The listing builds one solid part. Answer for the finished solid, in the listing's coordinates (mm). Face numbers are marked on the shaded views. A direction names the side the tool comes from. Round coordinates to 2 decimals unless told otherwise and drop trailing zeros. Loops run counter-clockwise (first coordinate to the right, second up) from the corner with the lowest first, then second, coordinate; pieces in that order, holes last. Notation, with made-up numbers: M -12.75,-19.5 L 5.25,-19.5 A32 cw 5.25,19.5 Z; hole C -18.5,19 d6. An arc over 180 degrees is marked long. Answer as a JSON object with one key per item and string values.
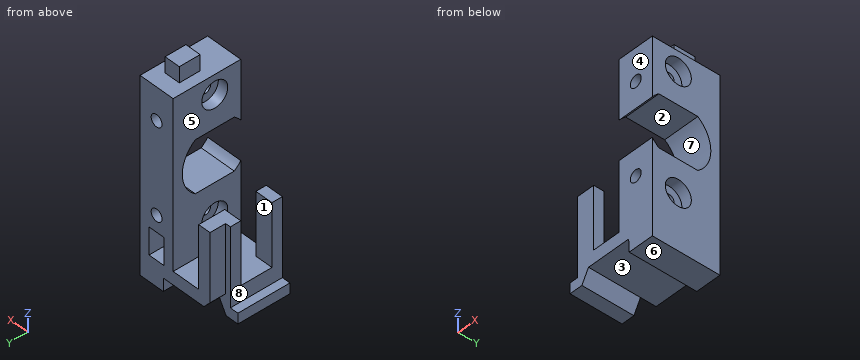
```python
from build123d import *

# Parameters (mm, degrees)
SKETCH2_R           = 1
BOSS_EXTRUDE1_DEPTH = 7
CUT_EXTRUDE1_START  = -5
SKETCH3_R           = 1.15
CUT_EXTRUDE1_DEPTH  = 13
SKETCH5_R           = 2.5
CUT_EXTRUDE2_DEPTH  = 2
CUT_EXTRUDE3_START  = 7
SKETCH5_2_R         = 2.5
CUT_EXTRUDE3_DEPTH  = 2
BOSS_EXTRUDE2_START = -5
BOSS_EXTRUDE2_DEPTH = 13
CUT_EXTRUDE4_START  = -5.4
SKETCH7_W           = 12
SKETCH7_H           = 6
CUT_EXTRUDE4_DEPTH  = 5
CUT_EXTRUDE5_START  = -10.4
SKETCH8_W           = 15
SKETCH8_H           = 13
CUT_EXTRUDE5_DEPTH  = 1.6
CUT_EXTRUDE6_START  = -8.8
SKETCH9_W           = 13
SKETCH9_H           = 3
CUT_EXTRUDE6_DEPTH  = 1
BOSS_EXTRUDE4_START = 8
SKETCH10_W          = 5.4
SKETCH10_H          = 5
BOSS_EXTRUDE4_DEPTH = 13
CUT_EXTRUDE7_START  = 8
SKETCH11_W          = 17.4
SKETCH11_H          = 3
CUT_EXTRUDE7_DEPTH  = 13
BOSS_EXTRUDE5_START = 15
SKETCH12_W          = 3
SKETCH12_H          = 4
BOSS_EXTRUDE5_DEPTH = 3
CUT_EXTRUDE8_START  = 8
CUT_EXTRUDE8_DEPTH  = 13
CUT_EXTRUDE9_START  = 8
CUT_EXTRUDE9_DEPTH  = 3
CUT_EXTRUDE10_START = 8
SKETCH15_W          = 3.2
SKETCH15_H          = 5.2
CUT_EXTRUDE10_DEPTH = 3.2


with BuildPart() as part:
    # Sketch2 → Boss-Extrude1 (new body)
    with BuildSketch(Plane(origin=(0, 0, 0), x_dir=(0, 0, -1), z_dir=(1, 0, 0))):
        with BuildLine():
            Line((3.75, -5), (15, -5))
            Line((15, -5), (15, 8))
            Line((15, 8), (-15, 8))
            Line((-15, 8), (-15, -5))
            Line((-15, -5), (-3.75, -5))
            ThreePointArc((-3.75, -5), (-4.419417382, -4.419417382), (-5, -3.75))
            Line((-5, -3.75), (-5, 3.75))
            ThreePointArc((-5, 3.75), (0, 6.25), (5, 3.75))
            Line((5, 3.75), (5, -3.75))
            ThreePointArc((5, -3.75), (4.419417382, -4.419417382), (3.75, -5))
        make_face()
        with Locations((-11.25, 0)):
            Circle(SKETCH2_R, mode=Mode.SUBTRACT)
        with Locations((11.25, 0)):
            Circle(SKETCH2_R, mode=Mode.SUBTRACT)
    extrude(amount=BOSS_EXTRUDE1_DEPTH)

    # Sketch3 → Cut-Extrude1 (cut)
    with BuildSketch(Plane(origin=(0, 0, 0), x_dir=(1, 0, 0), z_dir=(0, 1, 0)).offset(CUT_EXTRUDE1_START)):
        with Locations((3.5, 8.75)):
            Circle(SKETCH3_R)
        with Locations((3.5, -8.75)):
            Circle(SKETCH3_R)
    extrude(amount=CUT_EXTRUDE1_DEPTH, mode=Mode.SUBTRACT)

    # Sketch5 → Cut-Extrude2 (cut)
    with BuildSketch(Plane(origin=(0, 0, 0), x_dir=(0, 0, -1), z_dir=(1, 0, 0))):
        with Locations((11.25, 0)):
            Circle(SKETCH5_R)
        with Locations((-11.25, 0)):
            Circle(SKETCH5_R)
    extrude(amount=CUT_EXTRUDE2_DEPTH, mode=Mode.SUBTRACT)

    # Sketch5<2> → Cut-Extrude3 (cut)
    with BuildSketch(Plane(origin=(0, 0, 0), x_dir=(0, 0, -1), z_dir=(1, 0, 0)).offset(CUT_EXTRUDE3_START)):
        with Locations((11.25, 0)):
            Circle(SKETCH5_2_R)
        with Locations((-11.25, 0)):
            Circle(SKETCH5_2_R)
    extrude(amount=-CUT_EXTRUDE3_DEPTH, mode=Mode.SUBTRACT)

    # Sketch6 → Boss-Extrude2 (add)
    with BuildSketch(Plane(origin=(0, 0, 0), x_dir=(1, 0, 0), z_dir=(0, 1, 0)).offset(BOSS_EXTRUDE2_START)):
        Polygon((7, 15), (7, 25), (-10.4, 25), (-10.4, 5), (-5.4, 5), (-5.4, 22), (0, 22), (0, 15), align=None)
    extrude(amount=BOSS_EXTRUDE2_DEPTH)

    # Sketch7 → Cut-Extrude4 (cut)
    with BuildSketch(Plane(origin=(0, 0, 0), x_dir=(0, 0, -1), z_dir=(1, 0, 0)).offset(CUT_EXTRUDE4_START)):
        with Locations((11, 0)):
            Rectangle(SKETCH7_W, SKETCH7_H)
    extrude(amount=-CUT_EXTRUDE4_DEPTH, mode=Mode.SUBTRACT)

    # Sketch8 → Cut-Extrude5 (cut)
    with BuildSketch(Plane(origin=(0, 0, 0), x_dir=(0, 0, -1), z_dir=(1, 0, 0)).offset(CUT_EXTRUDE5_START)):
        with Locations((12.5, 1.5)):
            Rectangle(SKETCH8_W, SKETCH8_H)
    extrude(amount=CUT_EXTRUDE5_DEPTH, mode=Mode.SUBTRACT)

    # Sketch9 → Cut-Extrude6 (cut)
    with BuildSketch(Plane(origin=(0, 0, 0), x_dir=(0, 0, -1), z_dir=(1, 0, 0)).offset(CUT_EXTRUDE6_START)):
        with Locations((11.5, 6.5)):
            Rectangle(SKETCH9_W, SKETCH9_H)
    extrude(amount=CUT_EXTRUDE6_DEPTH, mode=Mode.SUBTRACT)

    # Sketch10 → Boss-Extrude4 (add)
    with BuildSketch(Plane(origin=(0, 0, 0), x_dir=(1, 0, 0), z_dir=(0, 1, 0)).offset(BOSS_EXTRUDE4_START)):
        with Locations((-2.7, 19.5)):
            Rectangle(SKETCH10_W, SKETCH10_H)
    extrude(amount=-BOSS_EXTRUDE4_DEPTH)

    # Sketch11 → Cut-Extrude7 (cut)
    with BuildSketch(Plane(origin=(0, 0, 0), x_dir=(1, 0, 0), z_dir=(0, 1, 0)).offset(CUT_EXTRUDE7_START)):
        with Locations((-1.7, 23.5)):
            Rectangle(SKETCH11_W, SKETCH11_H)
    extrude(amount=-CUT_EXTRUDE7_DEPTH, mode=Mode.SUBTRACT)

    # Sketch12 → Boss-Extrude5 (add)
    with BuildSketch(Plane.XY.offset(BOSS_EXTRUDE5_START)):
        with Locations((3.5, 3)):
            Rectangle(SKETCH12_W, SKETCH12_H)
    extrude(amount=BOSS_EXTRUDE5_DEPTH)

    # Sketch13 → Cut-Extrude8 (cut)
    with BuildSketch(Plane(origin=(0, 0, 0), x_dir=(1, 0, 0), z_dir=(0, 1, 0)).offset(CUT_EXTRUDE8_START)):
        Polygon((2.1, 22), (2.000079904, 19.501997603), (-6.499920096, 19.501997603), (-7.9, 22), align=None)
    extrude(amount=-CUT_EXTRUDE8_DEPTH, mode=Mode.SUBTRACT)

    # Sketch14 → Cut-Extrude9 (cut)
    with BuildSketch(Plane(origin=(0, 0, 0), x_dir=(1, 0, 0), z_dir=(0, 1, 0)).offset(CUT_EXTRUDE9_START)):
        Polygon((-6.499920096, 19.501997603), (-7.8, 18), (-8.8, 18), (-8.8, 20), (-10.4, 20), (-10.4, 22), (-7.9, 22), align=None)
    extrude(amount=-CUT_EXTRUDE9_DEPTH, mode=Mode.SUBTRACT)

    # Sketch15 → Cut-Extrude10 (cut)
    with BuildSketch(Plane(origin=(0, 0, 0), x_dir=(1, 0, 0), z_dir=(0, 1, 0)).offset(CUT_EXTRUDE10_START)):
        with Locations((3.5, 14.5)):
            Rectangle(SKETCH15_W, SKETCH15_H)
    extrude(amount=-CUT_EXTRUDE10_DEPTH, mode=Mode.SUBTRACT)


solid = part.part
```
Item 1: The part is cut by section D-D (z = 8). Give the vertices of the cut face in (x, y).
Values follow:
{"outline": "M 0,-5 L 2.63,-5 L 2.63,8 L 0,8 Z; M 4.37,-5 L 7,-5 L 7,8 L 4.37,8 Z"}
Item 2: Determine the mould class of the marked faces 6, 7 and 8 for opening direction Z: released by +Z, released by -Z, zero draft, split by the parting line, or undercut.
Values follow:
{"face 6": "released by -Z", "face 7": "undercut", "face 8": "zero draft"}
Item 3: Which of the six approach directions +Z, -Z, +X, -X, +Y, -Y give full straight-line access (tool end or side, diameter ignored) to the marked faces 1, 2, 3, 4 and 5?
Values follow:
{"face 1": "+Z, -X", "face 2": "+X, -X", "face 3": "-Z, +Y, -Y", "face 4": "+Z, -Z, +X, -X, -Y", "face 5": "+Z, +Y, -Y"}
Item 4: The part is cut by section A-A (y = -1.5). Give the number of separate pieces and of enclosed holes in the cut face, then the cut area to 3 significant figures.
Values follow:
{"separate pieces": "2", "enclosed holes": "2", "area": "173 mm^2"}
Item 5: The part is cut by section C-C (z = -11.25). Give the vertices of the cut face in (x, y), then the cut area to 3 significant figures.
Values follow:
{"outline": "M -8.8,-5 L -5.4,-5 L -5.4,-3 L -8.8,-3 Z; M -8.8,3 L -5.4,3 L -5.4,8 L -7.8,8 L -7.8,5 L -8.8,5 Z; M 0,-5 L 7,-5 L 7,-2.5 L 5,-2.5 L 5,-1 L 2,-1 L 2,-2.5 L 0,-2.5 Z; M 0,2.5 L 2,2.5 L 2,1 L 5,1 L 5,2.5 L 7,2.5 L 7,8 L 0,8 Z", "area": "85.8 mm^2"}
Item 6: Flat-ended cylindrical pins translate along their axes: P1, Ø6, axis at x = -5, y = -1.5, coming from the +Z side; P2, Ø5.5, axis at y = 1, z = -11.5, coming from the -X side; P3, Ø3, axis at y = 0, z = -11.25, coming from the +X side. Find the tip coordinate at first contact, or state that the pin passes through.
Values follow:
{"P1": "z = -5", "P2": "x = -8.8", "P3": "x = 5"}
Item 7: Straight lines are drawn through the part: line 1 (Z direction, x = 3.65, y = 0); line 2 (Z direction, x = 3.5, y = 2); line 3 (Y direction, x = 5.7, z = 11.25). For each, find the intervals that lie inside material, in ascending order.
Values follow:
{"line 1": "-22 to -12.25, -10.25 to -9.89, -7.61 to -5, 5 to 7.61, 9.89 to 10.25, 12.25 to 15", "line 2": "-22 to -9.9, -7.6 to -5, 5 to 7.6, 9.9 to 18", "line 3": "-5 to -2.5, 2.5 to 8"}
Item 8: The part is cut by section B-B (x = 3.5). Give the vertices of the cut face in (y, z).
Values follow:
{"outline": "M -5,-22 L 8,-22 L 8,-17.1 L 4.8,-17.1 L 4.8,-11.9 L 8,-11.9 L 8,-9.9 L -5,-9.9 Z; M -5,-7.6 L 8,-7.6 L 8,7.6 L -5,7.6 L -5,3.75 A6.25 cw -3.75,5 L 3.75,5 A6.25 cw 3.75,-5 L -3.75,-5 A6.25 cw -5,-3.75 Z; M -5,9.9 L 8,9.9 L 8,15 L 5,15 L 5,18 L 1,18 L 1,15 L -5,15 Z; hole C 0,-11.25 d2; hole C 0,11.25 d2"}
